Design review of the part built by this model. Coordinates are the model's own, in mm. A direction names the side the tool comes from. Coordinates: 2 decimals unless noted, no trailing zeros. Loops run counter-clockwise (first coordinate to the right, second up) from the corner with the lowest first, then second, coordinate; pieces in that order, holes last. Notation, with made-up numbers: M 83,-2 L 93,-2 A30 ccw 93,24 Z; hole C 27,-37 d2. An arc over 180 degrees is marked long. Put each result on its own line as item: value. Start each with the question number.
(1) Take a section at D-D, the plane y = 10. Give the boundary of the cut face in (x, z).
(2) The part is to be moulded in two halves that separate along X. For faces 3 (the flat face through (19.05, 2, 13)), 4 (the cylindrical face through (4.75, 1.5, 5.17)), 5 (the flat face through (9, 0, 13)), say which applies: +X half, -X half, draft (parallel to the pull), parting line (faces both ways), or undercut.
(3) Take a section at B-B, the plane x = 6.25. Give the boundary of the cut face in (y, z).
(4) Clearance check with flat-ended pins moving along their axes: pin 1 (3 mm diameter, centred on x = 6, z = 4.65, fed in from +Y); pin 2 (5 mm diameter, centred on y = 10, z = 13, fed in from +X); pin 3 (2 mm diameter, centred on y = 9.525, z = 5.08, fed in from -X). State where each tip first meets the part, or that it passes through.
(5) Take a section at A-A, the plane z = 20.32. Give the boundary of the cut face in (x, y).
(6) For probe 1 along Z at (x, y) = (6, 2.1); probe 2 along X at (y, z) = (1.8, 4.65); probe 3 along Y at (x, z) = (5.5, 19.25), list the stretches that pass through material, from the lowest coordinate up. Write a range as [from, to].
(7) For faces 1 (the cylindrical face through (5.38, 1.5, 21.85)), 2 (the flat face through (11, 3.048, 13)), list the 3-axis set-ups (+Z, -Z, +X, -X, +Y, -Y) from which the entire face can be reached by the end or side of a thin tool; tool diameter is ignored.
(8) Take a section at C-C, the plane y = 1.5. Give the boundary of the cut face in (x, z), then the cut area to 3 significant figures.
```python
from build123d import *

# Parameters (mm, degrees)
BOSS_EXTRUDE1_DEPTH   = 25.4
F_6_32_TAPPED_HOLE1_D = 2.7051
F_6_32_TAPPED_HOLE2_D = 2.7051


with BuildPart() as part:
    # Sketch1 → Boss-Extrude1 (new body)
    with BuildSketch(Plane.XY):
        Polygon((0, 0), (19.05, 0), (19.05, 3.048), (3.048, 3.048), (3.048, 19.05), (0, 19.05), align=None)
    extrude(amount=BOSS_EXTRUDE1_DEPTH)

    # #6-32 Tapped Hole1 (through all)
    with Locations(Plane(origin=(3.048, 0, 0), x_dir=(0, 0, -1), z_dir=(1, 0, 0))):
        with Locations((-20.32, 9.525), (-5.08, 9.525)):
            Hole(F_6_32_TAPPED_HOLE1_D / 2)

    # #6-32 Tapped Hole2 (through all)
    with Locations(Plane(origin=(0, 3.048, 0), x_dir=(1, 0, 0), z_dir=(0, 1, 0))):
        with Locations((6, -20.65), (6, -4.65)):
            Hole(F_6_32_TAPPED_HOLE2_D / 2)


solid = part.part
```
Computed values:
1. outline: M 0,0 L 3.05,0 L 3.05,3.81 L 0,3.81 Z; M 0,6.35 L 3.05,6.35 L 3.05,19.05 L 0,19.05 Z; M 0,21.59 L 3.05,21.59 L 3.05,25.4 L 0,25.4 Z
2. face 3: +X half
2. face 4: undercut
2. face 5: draft
3. outline: M 0,0 L 3.05,0 L 3.05,3.32 L 0,3.32 Z; M 0,5.98 L 3.05,5.98 L 3.05,19.32 L 0,19.32 Z; M 0,21.98 L 3.05,21.98 L 3.05,25.4 L 0,25.4 Z
4. pin 1: stops at y = 3.05
4. pin 2: stops at x = 3.05
4. pin 3: passes through
5. outline: M 0,0 L 4.69,0 L 4.69,3.05 L 3.05,3.05 L 3.05,8.17 L 0,8.17 Z; M 0,10.88 L 3.05,10.88 L 3.05,19.05 L 0,19.05 Z; M 7.31,0 L 19.05,0 L 19.05,3.05 L 7.31,3.05 Z
6. probe 1: z = [0, 3.3], [6, 19.3], [22, 25.4]
6. probe 2: x = [0, 4.65], [7.35, 19.05]
6. probe 3: y = [0, 3.05]
7. face 1: +Y, -Y
7. face 2: +Z, -Z, +X, +Y
8. outline: M 0,0 L 19.05,0 L 19.05,25.4 L 0,25.4 Z; hole C 6,4.65 d2.71; hole C 6,20.65 d2.71
8. area: 472 mm^2
